The listing builds one solid part. Answer for the finished solid, in the listing's coordinates (mm). Face numbers are marked on the shaded views. A direction names the side the tool comes from. Give positions to 0.01 mm unless a question says otherwise; leave off trailing zeros. Loops run counter-clockwise (first coordinate to the right, second up) from the corner with the lowest first, then second, coordinate; pieces in that order, holes last.
Item 1: Section C-C, the plane z = -9 is taken. Give the vertices of the cut face in (x, y) (3 decimals), and give its area (3 significant figures).
Item 2: A tool of negligible diameter and unlimited length cuts with its end or side. For the marked faces 1 and 2, from which of +Z, -Z, +X, -X, +Y, -Y can it reach the whole face along a straight path? Write none if from no direction.
Item 3: Section A-A, the plane y = 50 is taken. Give the vertices of the cut face in (x, z) (3 decimals), and give its area (3 significant figures).
Item 4: Consider line 1 along Y through (x, z) = (76, 23) (3 decimals); line 2 along X through (y, z) = (5, 23); line 3 along X through (y, z) = (127, 23). Determine where each line is inside the solid, lowest interval first.
Item 5: Each of these flat-tipped pins is pushed along its axis until it touches: pin 1 Ø2 at (x, y) = (-76.2, 34.925) entering from -Z; pin 2 Ø5.5 at (x, z) = (-1.29, -52.9) entering from +Y (3 decimals); pin 3 Ø2.5 at (x, z) = (-94, 23.5) entering from -Y (3 decimals); pin 4 Ø3 at (y, z) = (-21, -11.5) entering from -X. Where does it stop, or does it pass through?
Item 6: Section B-B, the plane x = -51.5 is taken. Give the vertices of the cut face in (y, z) (3 decimals), and give its area (3 significant figures).
from build123d import *

# Parameters (mm, degrees)
BASE_FLANGE1_DEPTH              = 102.87
SKETCH6_W                       = 9.525
SKETCH6_H                       = 99.06
CUT_EXTRUDE1_DEPTH              = 12.7
FILLET1_R                       = 21.336
FILLET2_R                       = 12.7
SKETCH8_W                       = 177.8
SKETCH8_H                       = 66.675
CUT_EXTRUDE2_DEPTH              = 10.16
F_27_0_144_DIAMETER_HOLE1_D     = 3.6576
F_27_0_144_DIAMETER_HOLE2_D     = 3.6576
CUT_EXTRUDE3_REACH              = 210.856
SKETCH17_R                      = 1.6
SKETCH17_W                      = 22.86
SKETCH17_H                      = 17.15
CUT_EXTRUDE4_REACH              = 210.856
SKETCH18_R                      = 5.5499
F_9_64_0_14063_DIAMETER_HOLE1_D = 3.572002


# Sheet-metal steps are written as plain solids
with BuildPart() as part:
    # Sketch1 → Base-Flange1 (new, symmetric)
    with BuildSketch(Plane.YZ):
        with BuildLine():
            Line((-25.4, -73.66), (-25.4, 15.875))
            ThreePointArc((-25.4, 15.875), (-22.610192091, 22.610192091), (-15.875, 25.4))
            Line((-15.875, 25.4), (152.4, 25.4))
            Line((152.4, 25.4), (152.4, 22.225))
            Line((152.4, 22.225), (-15.875, 22.225))
            ThreePointArc((-15.875, 22.225), (-20.365128061, 20.365128061), (-22.225, 15.875))
            Line((-22.225, 15.875), (-22.225, -73.66))
            Line((-22.225, -73.66), (-25.4, -73.66))
        make_face()
    extrude(amount=BASE_FLANGE1_DEPTH, both=True)

    # Sketch6 → Cut-Extrude1 (cut)
    with BuildSketch(Plane.YZ.offset(102.87)):
        with Locations((-20.6375, -24.13)):
            Rectangle(SKETCH6_W, SKETCH6_H)
    cut_extrude1 = extrude(amount=-CUT_EXTRUDE1_DEPTH, mode=Mode.SUBTRACT)

    # Mirror1: Cut-Extrude1 across plane
    add(cut_extrude1.mirror(Plane(origin=(0, 0, 0), x_dir=(0, 0, 1), z_dir=(1, 0, 0))), mode=Mode.SUBTRACT)

    # Fillet1
    fillet1_edges = [part.edges().sort_by_distance(p)[0] for p in [
        (102.87, 152.4, 23.8125),
        (-102.87, 152.4, 23.8125),
    ]]
    fillet(fillet1_edges, radius=FILLET1_R)

    # Fillet2
    fillet2_edges = [part.edges().sort_by_distance(p)[0] for p in [
        (90.17, -23.8125, -73.66),
        (-90.17, -23.8125, -73.66),
    ]]
    fillet(fillet2_edges, radius=FILLET2_R)

    # Sketch8 → Cut-Extrude2 (cut)
    with BuildSketch(Plane.XY.offset(25.4)):
        with Locations((0, 80.9625)):
            Rectangle(SKETCH8_W, SKETCH8_H)
    extrude(amount=-CUT_EXTRUDE2_DEPTH, mode=Mode.SUBTRACT)

    # #27 (0.144) Diameter Hole1 (through all)
    with Locations(Plane.XY.offset(25.4)):
        with Locations((-76.2, 127), (0, 127), (76.2, 127), (76.2, 34.925), (0, 34.925), (-76.2, 34.925)):
            Hole(F_27_0_144_DIAMETER_HOLE1_D / 2)

    # #27 (0.144) Diameter Hole2 (through all)
    with Locations(Plane.XY.offset(25.4)):
        with Locations((92.4814, 141.7574), (95.4278, 73.533), (95.4278, -25.273), (-95.758, -18.034), (-95.758, 66.294), (-92.3544, 141.351), (3.2512, 144.5768)):
            Hole(F_27_0_144_DIAMETER_HOLE2_D / 2)

    # Sketch17 → Cut-Extrude3 (cut, up to next)
    with BuildSketch(Plane.XY.offset(25.4), mode=Mode.PRIVATE) as cut_extrude3_sk1:
        with Locations((-86.89, 5.4)):
            Circle(SKETCH17_R)
    cut_extrude3_tool1 = extrude(cut_extrude3_sk1.sketch, amount=-CUT_EXTRUDE3_REACH, mode=Mode.PRIVATE) & part.part
    # Sketch17 → Cut-Extrude3 (cut, up to next)
    with BuildSketch(Plane.XY.offset(25.4), mode=Mode.PRIVATE) as cut_extrude3_sk2:
        with Locations((-57.89, 5.4)):
            Circle(SKETCH17_R)
    cut_extrude3_tool2 = extrude(cut_extrude3_sk2.sketch, amount=-CUT_EXTRUDE3_REACH, mode=Mode.PRIVATE) & part.part
    # Sketch17 → Cut-Extrude3 (cut, up to next)
    with BuildSketch(Plane.XY.offset(25.4), mode=Mode.PRIVATE) as cut_extrude3_sk3:
        with Locations((-72.39, 5.4)):
            Rectangle(SKETCH17_W, SKETCH17_H)
    cut_extrude3_tool3 = extrude(cut_extrude3_sk3.sketch, amount=-CUT_EXTRUDE3_REACH, mode=Mode.PRIVATE) & part.part
    add(cut_extrude3_tool1.solids().sort_by_distance((-86.89, 5.4, 25.4))[0], mode=Mode.SUBTRACT)
    add(cut_extrude3_tool2.solids().sort_by_distance((-57.89, 5.4, 25.4))[0], mode=Mode.SUBTRACT)
    add(cut_extrude3_tool3.solids().sort_by_distance((-72.39, 5.4, 25.4))[0], mode=Mode.SUBTRACT)

    # Sketch18 → Cut-Extrude4 (cut, up to next)
    with BuildSketch(Plane.XY.offset(25.4), mode=Mode.PRIVATE) as cut_extrude4_sk1:
        with Locations((-39.37, 5.4)):
            Circle(SKETCH18_R)
    cut_extrude4_tool1 = extrude(cut_extrude4_sk1.sketch, amount=-CUT_EXTRUDE4_REACH, mode=Mode.PRIVATE) & part.part
    add(cut_extrude4_tool1.solids().sort_by_distance((-39.37, 5.4, 25.4))[0], mode=Mode.SUBTRACT)

    # 9/64 (0.14063) Diameter Hole1 (through all)
    with Locations(Plane(origin=(0, -22.225, 0), x_dir=(1, 0, 0), z_dir=(0, 1, 0))):
        with Locations((-1.292500082, 52.897499996), (69.407499996, 4.887500004)):
            Hole(F_9_64_0_14063_DIAMETER_HOLE1_D / 2)


solid = part.part
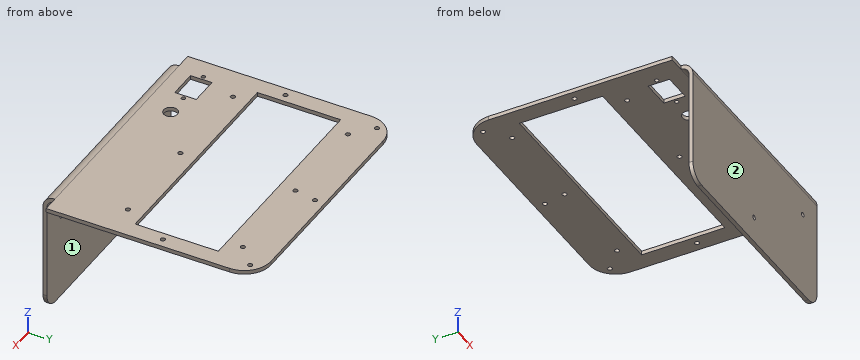
Worked answers:
1. outline: (-90.17, -25.4) - (90.17, -25.4) - (90.17, -22.225) - (-90.17, -22.225) - close
1. area: 573 mm2
2. face 1: -Z, +X, -X, +Y
2. face 2: +Z, -Z, +X, -X, -Y
3. outline: (-102.87, 22.225) - (-88.9, 22.225) - (-88.9, 25.4) - (-102.87, 25.4) - close; (88.9, 22.225) - (102.87, 22.225) - (102.87, 25.4) - (88.9, 25.4) - close
3. area: 88.7 mm2
4. line 1: y = -22.196 to 33.107, 36.743 to 47.625, 114.3 to 125.182, 128.818 to 152.4
4. line 2: x = -102.87 to -88.44, -85.34 to -83.82, -60.96 to -59.44, -56.34 to -44.91, -33.83 to 102.87
4. line 3: x = -102.87 to -78.03, -74.37 to -1.83, 1.83 to 74.37, 78.03 to 102.87
5. pin 1: passes through
5. pin 2: stops at y = -22.225
5. pin 3: stops at y = -15.875
5. pin 4: stops at x = -90.17
6. outline: (-25.4, -73.66) - (-22.225, -73.66) - (-22.225, 15.875) arc R6.35 cw to (-15.875, 22.225) - (47.625, 22.225) - (47.625, 25.4) - (-15.875, 25.4) arc R9.525 ccw to (-25.4, 15.875) - close; (114.3, 22.225) - (152.4, 22.225) - (152.4, 25.4) - (114.3, 25.4) - close
6. area: 646 mm2
